Autodesk Inventor part; units mm, degrees
ref_plane "YZ Plane" through (0, 0, 0) normal (1, 0, 0) x (0, 1, 0)
ref_plane "XZ Plane" through (0, 0, 0) normal (0, 1, 0) x (-1, 0, 0)
ref_plane "XY Plane" through (0, 0, 0) normal (0, 0, 1) x (1, 0, 0)
sketch "Sketch1" plane through (0, 0, 0) normal (0, 0, 1) x (1, 0, 0)
  circle A0 centre (29.8658, 2.0543) radius 1.1 construction
  circle A1 centre (-34.1342, 2.0543) radius 1.1 construction
  circle A2 centre (17.3658, -19.4457) radius 1.1 construction
  arc A3 (77.5658, -1.4457) -> (71.0658, 5.0543) centre (71.0658, -1.4457) ccw construction
  line L0 (-75.3342, 5.0543) -> (71.0658, 5.0543) construction
  arc A4 (-75.3342, 5.0543) -> (-81.8342, -1.4457) centre (-75.3342, -1.4457) ccw construction
  line L1 (-81.8342, -3.2457) -> (-81.8342, -1.4457) construction
  arc A5 (-81.8342, -3.2457) -> (-77.5665, -5.0135) centre (-79.3342, -3.2457) ccw construction
  line L2 (-75.4025, -2.8495) -> (-77.5665, -5.0135) construction
  arc A6 (-70.8063, -0.9457) -> (-75.4025, -2.8495) centre (-70.8063, -7.4457) ccw construction
  line L3 (7.8658, -0.9457) -> (-70.8063, -0.9457) construction
  arc A7 (14.3658, -7.4457) -> (7.8658, -0.9457) centre (7.8658, -7.4457) ccw construction
  line L4 (14.3658, -14.9457) -> (14.3658, -7.4457) construction
  line L5 (14.3658, -21.9457) -> (14.3658, -14.9457) construction
  line L6 (20.3658, -21.9457) -> (14.3658, -21.9457) construction
  line L7 (20.3658, -14.9457) -> (20.3658, -21.9457) construction
  line L8 (20.3658, -7.4457) -> (20.3658, -14.9457) construction
  arc A8 (26.8658, -0.9457) -> (20.3658, -7.4457) centre (26.8658, -7.4457) ccw construction
  line L9 (67.2302, -0.9457) -> (26.8658, -0.9457) construction
  arc A9 (69.7302, -1.4457) -> (67.2302, -0.9457) centre (67.2302, -7.4457) ccw construction
  line L10 (73.298, -5.0135) -> (69.7302, -1.4457) construction
  arc A10 (73.298, -5.0135) -> (77.5658, -3.2457) centre (75.0658, -3.2457) ccw construction
  line L11 (77.5658, -1.4457) -> (77.5658, -3.2457) construction
  circle A11 centre (17.3658, -15.6457) radius 0.75 construction
  circle A12 centre (-79.3342, -3.2457) radius 0.75 construction
  circle A13 centre (75.0658, -3.2457) radius 0.75 construction
  circle A14 centre (17.3658, -3.2457) radius 0.75 construction
  line L12 (-75.3342, 5.0543) -> (71.0658, 5.0543)
  line L13 (77.5658, -1.4457) -> (77.5658, -21.9457)
  line L14 (77.5658, -21.9457) -> (-81.8342, -21.9457)
  line L15 (-81.8342, -21.9457) -> (-81.8342, -1.4457)
  arc A15 (-75.3342, 5.0543) -> (-81.8342, -1.4457) centre (-75.3342, -1.4457) ccw
  arc A16 (77.5658, -1.4457) -> (71.0658, 5.0543) centre (71.0658, -1.4457) ccw
  point P0 (0, 0)
extrude "Extrusion1" add sketch "Sketch1" along normal blind 3
sketch "Sketch2" plane through (0, 0, 3) normal (0, 0, 1) x (1, 0, 0)
  circle A0 centre (29.8658, 2.0543) radius 1.1
  circle A1 centre (-34.1342, 2.0543) radius 1.1
  circle A2 centre (17.3658, -19.4457) radius 1.1
  point P0 (0, 0)
hole "Hole1" at (-34.1342, 2.0543, 3) at (17.3658, -19.4457, 3) at (29.8658, 2.0543, 3) direction (0, 0, -1) diameter 2.3 end through all counterbore diameter 4.5 counterbore depth 2.2
sketch "Sketch3" plane through (0, 0, 3) normal (0, 0, 1) x (1, 0, 0)
  line L0 (69.2331, -2.2265) -> (69.2331, -16.2835)
  line L1 (-61.3045, -16.2835) -> (-61.3045, -2.2265)
  circle A0 centre (-34.1342, 2.0543) radius 2.25 construction
  circle A1 centre (-34.1342, 2.0543) radius 1.15 construction
  circle A2 centre (29.8658, 2.0543) radius 2.25 construction
  circle A3 centre (29.8658, 2.0543) radius 1.15 construction
  circle A4 centre (17.3658, -19.4457) radius 2.25 construction
  circle A5 centre (17.3658, -19.4457) radius 1.15 construction
  arc A6 (-38.6902, 2.2735) -> (-29.7413, 1.5975) centre (-34.1902, 2.2735) ccw
  line L2 (-45.5022, 2.2735) -> (-38.6902, 2.2735)
  line L3 (-29.7413, 1.5975) -> (25.4168, 1.5975)
  line L4 (34.3147, 1.5975) -> (55.7139, 1.5975)
  arc A7 (25.4168, 1.5975) -> (34.3147, 1.5975) centre (29.8658, 2.2735) ccw
  line L5 (55.7139, -19.0025) -> (21.7425, -19.0025)
  line L6 (12.989, -19.0025) -> (-45.5022, -19.0025)
  arc A8 (21.7425, -19.0025) -> (12.989, -19.0025) centre (17.3658, -20.0483) ccw
  line L7 (-53.8342, -3.5957) -> (-53.8342, -15.2957)
  line L8 (-56.8342, -15.2957) -> (-56.8342, -3.5957)
  line L9 (-53.8342, -15.2957) -> (-56.8342, -15.2957)
  line L10 (-56.8342, -3.5957) -> (-53.8342, -3.5957)
  line L11 (63.8658, -15.5457) -> (63.8658, -3.3457)
  line L12 (66.6658, -3.3457) -> (66.6658, -15.5457)
  line L13 (66.6658, -15.5457) -> (63.8658, -15.5457)
  line L14 (63.8658, -3.3457) -> (66.6658, -3.3457)
  line L15 (-45.5022, 2.2735) -> (-45.5022, -2.2265)
  line L16 (-45.5022, -2.2265) -> (-61.3045, -2.2265)
  line L17 (-45.5022, -16.2835) -> (-45.5022, -19.0025)
  line L18 (-45.5022, -16.2835) -> (-61.3045, -16.2835)
  line L19 (55.7139, 1.5975) -> (55.7139, -2.2265)
  line L20 (55.7139, -2.2265) -> (69.2331, -2.2265)
  line L21 (55.7139, -19.0025) -> (55.7139, -16.2835)
  line L22 (55.7139, -16.2835) -> (69.2331, -16.2835)
  point P0 (0, 0)
  dimension "d9" = 4.5
  dimension "d10" = 4.5
  dimension "d11" = 4.5
  dimension "d15" = 20.6
extrude "Extrusion2" cut sketch "Sketch3" against normal through all contours L0 L22 L21 L5 A8 L6 L17 L18 L1 L16 L15 L2 A6 L3 A7 L4 L19 L20 | L7 L9 L8 L10 | L11 L14 L12 L13
fillet "Fillet1" radius 7.75 2 edges at (-81.8342, -21.9457, 1.5) (77.5658, -21.9457, 1.5)
sketch "Sketch4" plane through (-75.3342, 5.0543, 0) normal (0, 1, 0) x (1, 0, 0)
  line L0 (44.0825, -3) -> (102.5284, -3)
  line L1 (102.5284, -3) -> (102.5284, -19)
  line L2 (102.5284, -19) -> (44.0825, -19)
  line L3 (44.0825, -19) -> (44.0825, -3)
  line L4 (146.4, -3) -> (0, -3)
  point P0 (75.3342, 0)
  dimension "d16" = 16
extrude "Extrusion3" add sketch "Sketch4" against normal blind 3
sketch "Sketch5" plane through (-74.0842, -21.9457, 0) normal (0, -1, 0) x (1, 0, 0)
  line L0 (143.9, 3) -> (143.9, 0)
  line L1 (0, 3) -> (143.9, 3)
  line L2 (0, 0) -> (0, 3)
  line L3 (0, 0) -> (143.9, 0)
  line L4 (0, 3) -> (143.9, 3)
  line L5 (101.2784, 19) -> (42.8325, 19)
  line L6 (38.0287, 3) -> (54.0287, 3)
  line L7 (54.0287, 3) -> (54.0287, 19)
  line L8 (54.0287, 19) -> (38.0287, 19)
  line L9 (38.0287, 19) -> (38.0287, 3)
  point P0 (74.0842, 0)
  point P1 (89.4899, 23)
  point P2 (57.4899, 23)
  dimension "d25" = 16
extrude "Extrusion4" add sketch "Sketch5" against normal blind 2.5 contours L1 L9 L8 L5 L7
fillet "Fillet3" radius 4 2 edges at (-31.2517, 3.5543, 19) (27.1942, 3.5543, 19)
fillet "Fillet4" radius 3.25 4 edges at (-61.3045, -2.2265, 1.5) (-61.3045, -16.2835, 1.5) (69.2331, -2.2265, 1.5) (69.2331, -16.2835, 1.5)
fillet "Fillet5" radius 6.5 2 edges at (-36.0555, -20.6957, 19) (-20.0555, -20.6957, 19)
sketch "Sketch7" plane through (-74.0842, -21.9457, 0) normal (0, -1, 0) x (1, 0, 0)
  point P0 (74.0842, 0)
  point P1 (46.0287, 12.8596)
  point P2 (95.4084, 8.91)
  point P3 (78.425, 12.9132)
hole "Hole2" at (-28.0555, -21.9457, 12.8596) at (21.3241, -21.9457, 8.91) at (4.3407, -21.9457, 12.9132) direction (0, 1, 0) diameter 3.2 end through all
properties part number "xtion_custom_heatsink_mount" material "PC/ABS Plastic"
Could you check a few things on this model? Use its own coordinates, in mm. A direction names the side the tool comes from. Round coordinates to 2 decimals unless told otherwise and drop trailing zeros. Write each loop counter-clockwise with the first axis right and the second up, starting at its lowest first coordinate (ties: lowest second). Pieces come first, ordered by that corner, then holes. Notation, with made-up numbers: (32, 33) - (68, 33) arc R15 cw to (68, 49) - close; hole circle Ø9 at (71.25, 81.5). An arc over 180 degrees is marked (long way). Put each result on its own line as item: value. Start each with the question number.
(1) I want a section at A-A, the plane x = 64.5. Please give me the cut outline in (y, z), plus the area to 3 significant figures.
(2) Thinking about a two-plate mould opening in Y: for faces 1 (the cylindrical face through (75.61, 3.2, 1.48)), 2 (the flat face through (39, -19.002, 2)), 3 (the flat face through (-20.056, -21, 8)), which applies, released by +Y, released by -Y, zero draft, split by the parting line, or undercut?
(3) I need wall thicknesses on probe 1 along X at (y, z) = (-13.5, 2.5); probe 2 along Z at (x, y) = (36, 2.5); probe 3 along X at (y, z) = (-20.5, 12.5). Which ranges of each line are inside material? Lowest first, please.
(4) I want a section at C-C, the plane x = 9.5. Please give me the cut outline in (y, z), plus the area to 3 significant figures.
(5) I want a section at B-B, the plane z = 5. Please give me the cut outline in (x, y), plus the area to 3 significant figures.
(6) Will these pins go through, and if not, where does the flat tip stop? pin 1 (3 mm diameter, centred on x = -65.5, y = -15, fed in from +Z); pin 2 (2.5 mm diameter, centred on y = 0.5, z = 2, fed in from -X); pin 3 (3.5 mm diameter, centred on x = 29.87, y = 2.05, fed in from +Z).
(7) I want a section at D-D, the plane x = -66.5. Please give me the cut outline in (y, z).
(8) For faces 4 (the flat face through (-28, -19.446, 11)), 5 (the cylindrical face through (-36, 0.8, 1.9)), 6 (the flat face through (55.714, 0, 2)), which set-ups out of +Z, -Z, +X, -X, +Y, -Y let a thin tool reach every point of the face, with its end or its side?
Here are the results:
1. outline: (-21.95, 0) - (-16.28, 0) - (-16.28, 3) - (-21.95, 3) - close; (-2.23, 0) - (5.05, 0) - (5.05, 3) - (-2.23, 3) - close
1. area: 38.8 mm^2
2. face 1: released by +Y
2. face 2: undercut
2. face 3: zero draft
3. probe 1: x = -81.83 to -61.27, 69.2 to 77.57
3. probe 2: z = 0 to 3
3. probe 3: x = -36.06 to -29.61, -26.5 to -20.06
4. outline: (-21.95, 0) - (-19, 0) - (-19, 3) - (-21.95, 3) - close; (1.6, 0) - (5.05, 0) - (5.05, 19) - (2.05, 19) - (2.05, 3) - (1.6, 3) - close
4. area: 67.2 mm^2
5. outline: (-36.06, -21.95) - (-20.06, -21.95) - (-20.06, -19.45) - (-36.06, -19.45) - close; (-31.25, 2.05) - (27.19, 2.05) - (27.19, 5.05) - (-31.25, 5.05) - close
5. area: 215 mm^2
6. pin 1: stops at z = 3
6. pin 2: stops at x = -81.8
6. pin 3: stops at z = 0.8
7. outline: (-21.95, 0) - (5.05, 0) - (5.05, 3) - (-21.95, 3) - close
8. face 4: +Z, +X, -X
8. face 5: +Z
8. face 6: +Z, -Z
